Geometry: final body of the model. Coordinates: model frame, mm. A direction names the side the tool comes from. Round coordinates to 2 decimals unless told otherwise and drop trailing zeros. Order: outer loops, then holes, each group sorted by start corner. A loop starts at its lowest first (then second) coordinate and runs counter-clockwise, first axis right, second up. Notation, with made-up numbers: (69, -24) -> (90, -24) arc R18 cw to (90, -9) -> close; hole circle Ø4 at (34.5, 6). An arc over 180 degrees is marked (long way). Put each result on its own line as item: value.
```python
from build123d import *

# Parameters (mm, degrees)
SKETCH1_W           = 150
SKETCH1_H           = 48
SKETCH1_R           = 4.1
BOSS_EXTRUDE1_DEPTH = 5
BOSS_EXTRUDE2_DEPTH = 20
BOSS_EXTRUDE3_DEPTH = 25
BOSS_EXTRUDE4_START = -150
BOSS_EXTRUDE4_DEPTH = 25
BOSS_EXTRUDE5_START = -75
BOSS_EXTRUDE5_DEPTH = 32.5
FILLET5_SIZE        = 10
FILLET5_SIZE_2      = 4
FILLET6_SIZE        = 10
FILLET6_SIZE_2      = 4


with BuildPart() as part:
    # Sketch1 → Boss-Extrude1 (new body)
    with BuildSketch(Plane.XY):
        with Locations((0, 24)):
            Rectangle(SKETCH1_W, SKETCH1_H)
        with Locations((-41, 10)):
            Circle(SKETCH1_R, mode=Mode.SUBTRACT)
        with Locations((41, 10)):
            Circle(SKETCH1_R, mode=Mode.SUBTRACT)
    extrude(amount=BOSS_EXTRUDE1_DEPTH)

    # Sketch2 → Boss-Extrude2 (add)
    with BuildSketch(Plane.XY):
        with BuildLine():
            Line((-75, 5), (-75, 0))
            Line((-75, 0), (75, 0))
            Line((75, 0), (75, 5))
            Line((75, 5), (48.5, 5))
            add(Edge.make_bspline(
                [(33.5, 5), (36.476810307, 4.895138539), (41.670990079, -0.895128503), (44.181209535, 4.895118466), (48.5, 5)],
                knots=[0, 0, 0, 0, 0.5, 1, 1, 1, 1], degree=3))
            Line((33.5, 5), (-33.5, 5))
            add(Edge.make_bspline(
                [(-48.5, 5), (-45.523189693, 4.895138539), (-40.329009921, -0.895128503), (-37.818790465, 4.895118466), (-33.5, 5)],
                knots=[0, 0, 0, 0, 0.5, 1, 1, 1, 1], degree=3))
            Line((-48.5, 5), (-75, 5))
        make_face()
    extrude(amount=BOSS_EXTRUDE2_DEPTH)

    # Sketch4 → Boss-Extrude3 (add)
    with BuildSketch(Plane.ZY.offset(75)):
        Polygon((5, 5), (12.5, 5), (5, 15), align=None)
    extrude(amount=-BOSS_EXTRUDE3_DEPTH)

    # Sketch4<2> → Boss-Extrude4 (add)
    with BuildSketch(Plane.ZY.offset(75).offset(BOSS_EXTRUDE4_START)):
        Polygon((5, 5), (12.5, 5), (5, 15), align=None)
    extrude(amount=BOSS_EXTRUDE4_DEPTH)

    # Sketch4<3> → Boss-Extrude5 (add, symmetric)
    with BuildSketch(Plane.ZY.offset(75).offset(BOSS_EXTRUDE5_START)):
        Polygon((5, 5), (12.5, 5), (5, 15), align=None)
    extrude(amount=BOSS_EXTRUDE5_DEPTH, both=True)

    # Fillet5
    # an asymmetric fillet: 10, 4 mm, written as the material it takes off along each edge
    with BuildSketch(Plane(origin=(-75, 0, 45), x_dir=(1, 0, 0), z_dir=(0, 0, -1))) as fillet5_piece_1:
        with BuildLine():
            Bezier((FILLET5_SIZE, 0), (0, 0), (0, -FILLET5_SIZE_2), weights=[1, 0.707106781, 1])
            Line((0, -FILLET5_SIZE_2), (0, 0))
            Line((0, 0), (FILLET5_SIZE, 0))
        make_face()
    extrude(amount=70, mode=Mode.SUBTRACT)

    # Fillet6
    # an asymmetric fillet: 10, 4 mm, written as the material it takes off along each edge
    with BuildSketch(Plane(origin=(75, 0, -25), x_dir=(-1, 0, 0), z_dir=(0, 0, 1))) as fillet6_piece_1:
        with BuildLine():
            Bezier((FILLET6_SIZE, 0), (0, 0), (0, -FILLET6_SIZE_2), weights=[1, 0.707106781, 1])
            Line((0, -FILLET6_SIZE_2), (0, 0))
            Line((0, 0), (FILLET6_SIZE, 0))
        make_face()
    extrude(amount=70, mode=Mode.SUBTRACT)


solid = part.part
```
1. Contact query for flat-ended pins moving along their axis: P1, Ø4, axis at y = 19, z = 7.5, coming from the -X side; P2, Ø12, axis at x = 60.5, z = 11.5, coming from the +Y side; P3, Ø1, axis at x = 28.5, y = 32.5, coming from the +Z side; P4, Ø4.5, axis at x = 6.5, z = 10, coming from the +Y side. Output: stop coordinate, or through.
Ans:
P1: through
P2: y = 14.33
P3: z = 5
P4: y = 11.33
2. Set-up query: faces 1 (the face through (32.5, 8, 7)), 2 (the face through (-62.675, 9.93, 8.802)). Return all of +Z, -Z, +X, -X, +Y, -Y with unobstructed straight access to the full face (end or side cutting, diameter ignored); none if empty.
Ans:
face 1: +Z, +Y
face 2: +Z, +X, -X, +Y
3. Cut plane C-C on z = 2.5. State how many separate pieces and enclosed holes the cut face has, and give its area (3 significant figures).
Ans:
separate pieces: 1
enclosed holes: 2
area: 7,080 mm²
4. Material intervals for probe 1 along Y at (x, z) = (41, 2.95); probe 2 along Z at (x, y) = (23, 45); probe 3 along Y at (x, z) = (-41, 17.25), sorted ascending.
Ans:
probe 1: 0 to 5.9, 14.1 to 48
probe 2: 0 to 5
probe 3: 0 to 2
5. Cut plane A-A on y = 10. Return loops of the section in (x, z).
Ans:
outline: (-75, 0) -> (-45.1, 0) -> (-45.1, 5) -> (-50, 5) -> (-50, 8.75) -> (-75, 8.75) -> close; (-36.9, 0) -> (36.9, 0) -> (36.9, 5) -> (32.5, 5) -> (32.5, 8.75) -> (-32.5, 8.75) -> (-32.5, 5) -> (-36.9, 5) -> close; (45.1, 0) -> (75, 0) -> (75, 8.75) -> (50, 8.75) -> (50, 5) -> (45.1, 5) -> close
6. Draft query along X for faces 3 (the face through (-75, 23, 4)), 4 (the face through (36.904, 10.18, 2.465)), 5 (the face through (62.675, 9.93, 8.802)). Return one class per face: +X half, -X half, draft (parallel to the pull), parting line (faces both ways), or undercut.
Ans:
face 3: -X half
face 4: undercut
face 5: draft
7. Cut plane D-D on y = 17. Return loops of the section in (x, z).
Ans:
outline: (-75, 0) -> (75, 0) -> (75, 5) -> (-75, 5) -> close
8. Cut plane B-B on x = 22. Return loops of the section in (y, z).
Ans:
outline: (0, 0) -> (48, 0) -> (48, 5) -> (15, 5) -> (5, 12.5) -> (5, 20) -> (0, 20) -> close
